The listing builds one solid part. Answer for the finished solid, in the listing's coordinates (mm). A direction names the side the tool comes from. Round coordinates to 2 decimals unless told otherwise and drop trailing zeros. Order: outer loops, then holes, each group sorted by start corner. A loop starts at its lowest first (then second) coordinate and runs counter-clockwise, first axis right, second up. Notation, with made-up numbers: (9, -34.5) -> (55, -34.5) arc R9 ccw to (55, -18.5) -> close; hole circle Ø3 at (24, -17). An arc over 180 degrees is marked (long way). Answer in a Markdown table with one row per item. Add a question column.
```python
from build123d import *

# Parameters (mm, degrees)
SKETCH_1_W          = 50
SKETCH_1_H          = 35
EXTRUDE_1_DEPTH     = 30
HOLE_WIZARD_345_D   = 8.5
HOLE_WIZARD_450_D   = 3.2
HOLE_WIZARD_604_D   = 15
CHAMFER_1_SIZE      = 1
CHAMFER_1_SIZE_2    = 0.708203932
HOLE_WIZARD_1_D     = 10.5
HOLE_WIZARD_1_DEPTH = 12


with BuildPart() as part:
    # 草图1 → 凸台-拉伸1 (new body)
    with BuildSketch(Plane.XY):
        Rectangle(SKETCH_1_W, SKETCH_1_H)
    extrude(amount=EXTRUDE_1_DEPTH)

    # Hole Wizard 345 (through all)
    with Locations(Plane.XY.offset(30)):
        with Locations((0, 0)):
            Hole(HOLE_WIZARD_345_D / 2)

    # Hole Wizard 450 (through all)
    with Locations(Plane.XY.offset(30)):
        with Locations((8, 0), (0, 8), (-8, 0), (0, -8)):
            Hole(HOLE_WIZARD_450_D / 2)

    # Hole Wizard 604 (through all)
    with Locations(Plane.XY.offset(30)):
        with Locations((20, 0), (-20, 0)):
            Hole(HOLE_WIZARD_604_D / 2)

    # 倒角1
    # the kernel refuses this chamfer: 1, 0.708203932 mm, written as the material it takes off along each edge
    with BuildSketch(Plane(origin=(-20, 0, 0), x_dir=(-0.8790200859122482, 0.4767847402789059, 0), z_dir=(-0.4767847402789059, -0.8790200859122482, 0))) as chamfer_1_piece_1:
        Polygon((7.5, -CHAMFER_1_SIZE), (7.5 + CHAMFER_1_SIZE, 0), (7.5, 0), align=None)
    revolve(axis=Axis((-20, 0, 0), (0, 0, -1)), revolution_arc=303.048763938, mode=Mode.SUBTRACT)
    with BuildSketch(Plane(origin=(-20, 0, 30), x_dir=(-0.879020085912248, 0.47678474027890627, 0), z_dir=(-0.47678474027890627, -0.879020085912248, 0))) as chamfer_1_piece_2:
        Polygon((7.5 + CHAMFER_1_SIZE, 0), (7.5, CHAMFER_1_SIZE), (7.5, 0), align=None)
    revolve(axis=Axis((-20, 0, 30), (0, 0, -1)), revolution_arc=303.048763938, mode=Mode.SUBTRACT)
    with BuildSketch(Plane(origin=(20, 0, 30), x_dir=(0.879020085912248, -0.4767847402789061, 0), z_dir=(0.4767847402789061, 0.879020085912248, 0))) as chamfer_1_piece_3:
        Polygon((7.5 + CHAMFER_1_SIZE, 0), (7.5, CHAMFER_1_SIZE), (7.5, 0), align=None)
    revolve(axis=Axis((20, 0, 30), (0, 0, -1)), revolution_arc=303.048763938, mode=Mode.SUBTRACT)
    with BuildSketch(Plane(origin=(20, 0, 0), x_dir=(0.8790200859122481, 0.476784740278906, 0), z_dir=(0.476784740278906, -0.8790200859122481, 0))) as chamfer_1_piece_4:
        Polygon((7.5, CHAMFER_1_SIZE), (7.5 + CHAMFER_1_SIZE, 0), (7.5, 0), align=None)
    revolve(axis=Axis((20, 0, 0), (0, 0, 1)), revolution_arc=303.048763938, mode=Mode.SUBTRACT)
    with BuildSketch(Plane(origin=(-25, 5.590169944, 32.778051389), x_dir=(0.7914486393779661, 0.611235675682274, 0), z_dir=(0, 0, -1)), Plane(origin=(25, -5.590169944, 32.778051389), x_dir=(-0.7914486393779661, -0.611235675682274, 0), z_dir=(0, 0, -1))) as chamfer_1_piece_5:
        with BuildLine():
            Line((1.080663788, 0), (CHAMFER_1_SIZE_2 * 0.611235676113, -CHAMFER_1_SIZE_2 * 0.791448639936))
            Line((CHAMFER_1_SIZE_2 * 0.611235676113, -CHAMFER_1_SIZE_2 * 0.791448639936), (0, 0))
            ThreePointArc((0, 0), (0.555522087, -0.019473843), (1.080663788, 0))
        make_face()
    extrude(amount=35.556102778, mode=Mode.SUBTRACT)
    with BuildSketch(Plane(origin=(-25, -5.590169944, 32.778051389), x_dir=(0.7914486393779665, -0.6112356756822735, 0), z_dir=(0, 0, -1))) as chamfer_1_piece_6:
        with BuildLine():
            Line((1.080663788, 0), (CHAMFER_1_SIZE_2 * 0.611235676113, CHAMFER_1_SIZE_2 * 0.791448639936))
            Line((CHAMFER_1_SIZE_2 * 0.611235676113, CHAMFER_1_SIZE_2 * 0.791448639936), (0, 0))
            ThreePointArc((0, 0), (0.555522087, 0.019473843), (1.080663788, 0))
        make_face()
    extrude(amount=35.556102778, mode=Mode.SUBTRACT)
    with BuildSketch(Plane(origin=(25, 5.590169944, 32.778051389), x_dir=(0, 1, 0), z_dir=(0, 0, -1))) as chamfer_1_piece_7:
        with BuildLine():
            Line((CHAMFER_1_SIZE_2, 0), (0.660540261, -0.855289885))
            ThreePointArc((0.660540261, -0.855289885), (0.354967464, -0.427764092), (0, 0))
            Line((0, 0), (CHAMFER_1_SIZE_2, 0))
        make_face()
    extrude(amount=35.556102778, mode=Mode.SUBTRACT)

    # 孔1
    with Locations(Plane(origin=(0, 0, 0), x_dir=(-1, 0, 0), z_dir=(0, 0, -1))):
        with Locations((0, 0)):
            Hole(HOLE_WIZARD_1_D / 2, depth=HOLE_WIZARD_1_DEPTH)


solid = part.part
```
1. This flat-tipped pin is pushed along its axis until it touches: pin 1 (2 mm diameter, centred on y = -5, z = 25.5, fed in from -X). Where does it stop, or does it pass through?
2. The part is cut by section B-B (z = 17). Give the vertices of the cut face in (x, y).
3. For faces 5 (the flat face through (0, 17.5, 15)), 6 (the flat face through (2, -4, 12)), determine the directions among +Z, -Z, +X, -X, +Y, -Y from which every point of the face is accessible in a straight line to the end or side of a thin tool.
4. The part is cut by section C-C (x = -8). Give the vertices of the cut face in (y, z), then the cut area to 3 significant figures.
5. The part is cut by section D-D (z = 3). Give the vertices of the cut face in (x, y), then the cut area to 3 significant figures.
6. Straight lines are drawn through the part: line 1 along Y through (x, z) = (20, 9.5); line 2 along X through (y, z) = (-1, 3); line 3 along Y through (x, z) = (3, 27.5). For each, find the intervals that lie inside material, in ascending order.
7. The mould has two halves that part along X. Classify faces 1 (the cylindrical face through (0.35, -9.56, 14.79)), 2 (the conical face through (12.3, -0.2, 29.2)), 3 (the flat face through (-25, -12, 15)), 4 (the flat face through (-6, 0, 0)): released by +X, released by -X, zero draft, split by the parting line, or undercut.
8. The part is cut by section A-A (x = -20). Give the vertices of the cut face in (y, z), then the cut area to 3 significant figures.
Report:
| question | item | result |
|---|---|---|
| 1 | pin 1 | stops at x = -15.5 |
| 2 | outline | (-25, -17.5) -> (25, -17.5) -> (25, -6.3) -> (24.14, -6.25) arc R7.5 cw (long way) to (24.14, 6.25) -> (25, 6.3) -> (25, 17.5) -> (-25, 17.5) -> (-25, 6.3) -> (-24.14, 6.25) arc R7.5 cw (long way) to (-24.14, -6.25) -> (-25, -6.3) -> close; hole circle Ø3.2 at (-8, 0); hole circle Ø8.5 at (0, 0); hole circle Ø3.2 at (0, -8); hole circle Ø3.2 at (0, 8); hole circle Ø3.2 at (8, 0) |
| 3 | face 5 | +Z, -Z, +X, -X, +Y |
| 3 | face 6 | -Z |
| 4 | outline | (-17.5, 0) -> (-1.6, 0) -> (-1.6, 30) -> (-17.5, 30) -> close; (1.6, 0) -> (17.5, 0) -> (17.5, 30) -> (1.6, 30) -> close |
| 4 | area | 954 mm^2 |
| 5 | outline | (-25, -17.5) -> (25, -17.5) -> (25, -6.3) -> (24.14, -6.25) arc R7.5 cw (long way) to (24.14, 6.25) -> (25, 6.3) -> (25, 17.5) -> (-25, 17.5) -> (-25, 6.3) -> (-24.14, 6.25) arc R7.5 cw (long way) to (-24.14, -6.25) -> (-25, -6.3) -> close; hole circle Ø3.2 at (-8, 0); hole circle Ø10.5 at (0, 0); hole circle Ø3.2 at (0, -8); hole circle Ø3.2 at (0, 8); hole circle Ø3.2 at (8, 0) |
| 5 | area | 1,320 mm^2 |
| 6 | line 1 | y = -17.5 to -7.5, 7.5 to 17.5 |
| 6 | line 2 | x = -12.57 to -9.25, -6.75 to -5.15, 5.15 to 6.75, 9.25 to 12.57 |
| 6 | line 3 | y = -17.5 to -3.01, 3.01 to 17.5 |
| 7 | face 1 | undercut |
| 7 | face 2 | undercut |
| 7 | face 3 | released by -X |
| 7 | face 4 | zero draft |
| 8 | outline | (-17.5, 0) -> (-8.5, 0) -> (-7.5, 1) -> (-7.5, 29) -> (-8.5, 30) -> (-17.5, 30) -> close; (7.5, 1) -> (8.5, 0) -> (17.5, 0) -> (17.5, 30) -> (8.5, 30) -> (7.5, 29) -> close |
| 8 | area | 598 mm^2 |
